from build123d import *

# Parameters (mm, degrees)
F1_DEPTH = 4.83
F2_W     = 0.46
F2_H     = 0.46
F3_DEPTH = 10


with BuildPart() as f1:
    # F0 (on Top) → F1 (new body)
    with BuildSketch(Plane.XY):
        with BuildLine():
            ThreePointArc((2.415, 0.635), (0, 2.497088), (-2.415, 0.635))
            Line((-2.415, 0.635), (-2.303889, -0.635))
            Line((-2.303889, -0.635), (2.303889, -0.635))
            Line((2.303889, -0.635), (2.415, 0.635))
        make_face()
    extrude(amount=F1_DEPTH)

    # F2 (on face) → F3 (join)
    with BuildSketch(Plane(origin=(0, 0, 0), x_dir=(1, 0, 0), z_dir=(0, 0, -1))):
        with Locations((0, -0.635)):
            Rectangle(F2_W, F2_H)
        with Locations((1.27, -0.635)):
            Rectangle(F2_W, F2_H)
        with Locations((-1.27, -0.635)):
            Rectangle(F2_W, F2_H)
    extrude(amount=F3_DEPTH)


solid = f1.part
For this review, take the finished solid that the model builds, in its own axes (mm). Round coordinates to 2 decimals unless told otherwise and drop trailing zeros. Write each loop counter-clockwise with the first axis right and the second up, starting at its lowest first coordinate (ties: lowest second). Pieces come first, ordered by that corner, then holes. Notation, with made-up numbers: (1, 48) -> (46, 48) arc R27 ccw to (46, 69) -> close; hole circle Ø1 at (-8.5, 29). An arc over 180 degrees is marked (long way). Put each result on its own line as item: value.
Q1. Consider section B-B on y = -0.15. State the section outline as (x, z) points, and give its area (3 significant figures).
Determined:
outline: (-2.35, 0) -> (2.35, 0) -> (2.35, 4.83) -> (-2.35, 4.83) -> close
area: 22.7 mm^2
Q2. Consider section A-A on z = -2.25. State the section outline as (x, y) points (3 decimals), and give its area (3 significant figures).
Determined:
outline: (-1.5, 0.405) -> (-1.04, 0.405) -> (-1.04, 0.865) -> (-1.5, 0.865) -> close; (-0.23, 0.405) -> (0.23, 0.405) -> (0.23, 0.865) -> (-0.23, 0.865) -> close; (1.04, 0.405) -> (1.5, 0.405) -> (1.5, 0.865) -> (1.04, 0.865) -> close
area: 0.635 mm^2
Q3. To check wall thickness, follow L1, parallel to X at y = 0.65, z = -6.25; L2, parallel to Z at x = -1.65, y = -0.3; L3, parallel to Y at x = -0.05, z = -5 (3 decimals). State the ranges of each line that lie inside material, in increasing order. Write a range as [from, to].
Determined:
L1: x = [-1.5, -1.04], [-0.23, 0.23], [1.04, 1.5]
L2: z = [0, 4.83]
L3: y = [0.405, 0.865]
Q4. Consider section C-C on z = 1. State the section outline as (x, y) points (3 decimals).
Determined:
outline: (-2.415, 0.635) -> (-2.304, -0.635) -> (2.304, -0.635) -> (2.415, 0.635) arc R2.497 ccw to start
Q5. Clearance check with flat-ended pins moving along their axes: pin 1 Ø1.5 at (x, y) = (-0.5, 1.5) entering from -Z; pin 2 Ø0.5 at (y, z) = (0.5, -4.5) entering from +X; pin 3 Ø0.5 at (x, z) = (1.5, -4) entering from +Y (3 decimals); pin 4 Ø0.5 at (x, z) = (-1.5, -7) entering from -Y (3 decimals). State where each tip first meets the part, or that it passes through.
Determined:
pin 1: stops at z = -10
pin 2: stops at x = 1.5
pin 3: stops at y = 0.865
pin 4: stops at y = 0.405
